Build history of the part. All positions in model axes, mm. Face numbers are marked on the shaded views. A direction names the side the tool comes from. Coordinates: 2 decimals unless noted, no trailing zeros. Loops run counter-clockwise (first coordinate to the right, second up) from the corner with the lowest first, then second, coordinate; pieces in that order, holes last. Notation, with made-up numbers: (-7, 37.25) - (10, 37.25) arc R27 ccw to (10, 56.25) - close; hole circle Ø10 at (-13.5, -31.5). An arc over 180 degrees is marked (long way). One line per item, written item: value.
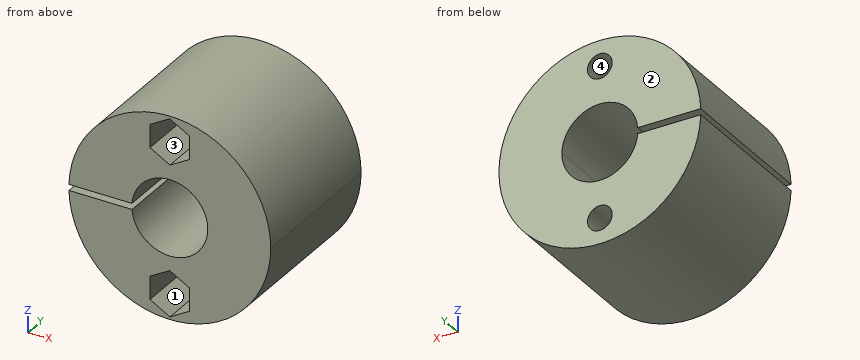
```python
from build123d import *

# Parameters (mm, degrees)
BOSS_EXTRUDE2_DEPTH = 50
CUT_EXTRUDE1_REACH  = 70.88
SKETCH3_R           = 4.1
CUT_EXTRUDE2_DEPTH  = 30


with BuildPart() as part:
    # Sketch2 → Boss-Extrude2 (new body)
    with BuildSketch(Plane(origin=(0, 0, 0), x_dir=(1, 0, 0), z_dir=(0, 1, 0))):
        with BuildLine():
            ThreePointArc((12.6, 0), (0.500394765, -12.590059773), (-12.560254774, -1))
            Line((-12.560254774, -1), (-33.485071301, -1))
            ThreePointArc((-33.485071301, -1), (0.500055713, -33.496267617), (33.5, 0))
            ThreePointArc((33.5, 0), (0.500055713, 33.496267617), (-33.485071301, 1))
            Line((-33.485071301, 1), (-12.560254774, 1))
            ThreePointArc((-12.560254774, 1), (0.500394765, 12.590059773), (12.6, 0))
        make_face()
    extrude(amount=BOSS_EXTRUDE2_DEPTH)

    # Sketch3 → Cut-Extrude1 (cut, up to next)
    with BuildSketch(Plane.XZ, mode=Mode.PRIVATE) as cut_extrude1_sk1:
        with Locations(Location((0, 25, 0), (0, 0, 270))):
            Circle(SKETCH3_R)
    cut_extrude1_tool1 = extrude(cut_extrude1_sk1.sketch, amount=-CUT_EXTRUDE1_REACH, mode=Mode.PRIVATE) & part.part
    # Sketch3 → Cut-Extrude1 (cut, up to next)
    with BuildSketch(Plane.XZ, mode=Mode.PRIVATE) as cut_extrude1_sk2:
        with Locations(Location((0, -25, 0), (0, 0, 270))):
            Circle(SKETCH3_R)
    cut_extrude1_tool2 = extrude(cut_extrude1_sk2.sketch, amount=-CUT_EXTRUDE1_REACH, mode=Mode.PRIVATE) & part.part
    add(cut_extrude1_tool1.solids().sort_by_distance((0, 0, 25))[0], mode=Mode.SUBTRACT)
    add(cut_extrude1_tool2.solids().sort_by_distance((0, 0, -25))[0], mode=Mode.SUBTRACT)

    # Sketch8 → Cut-Extrude2 (cut)
    with BuildSketch(Plane.XZ):
        Polygon((6.618426782, 21.22158407), (6.581417572, 28.842517761), (-0.03700921, 32.620933691), (-6.618426782, 28.77841593), (-6.581417572, 21.157482239), (0.03700921, 17.379066309), align=None)
        Polygon((6.618426782, -28.77841593), (6.581417572, -21.157482239), (-0.03700921, -17.379066309), (-6.618426782, -21.22158407), (-6.581417572, -28.842517761), (0.03700921, -32.620933691), align=None)
    extrude(amount=-CUT_EXTRUDE2_DEPTH, mode=Mode.SUBTRACT)


solid = part.part
```
Item 1: Cut at D-D, the plane z = 19. Write the cut outline in (x, y), then the cut area to 3 significant figures.
Check result:
outline: (-27.59, 0) - (-2.8, 0) - (-2.8, 30) - (2.81, 30) - (2.81, 0) - (27.59, 0) - (27.59, 50) - (-27.59, 50) - close
area: 2,590 mm^2
Item 2: Drop flat-ended pins along their axis: P1, Ø9.5, axis at x = 0, z = 25, coming from the -Y side; P2, Ø4, axis at y = 9, z = -4.5, coming from the +X side; P3, Ø6.5, axis at x = -19.5, y = 14, coming from the +Z side. Give the stop position or say it passes through.
Check result:
P1: stops at y = 30
P2: stops at x = 33.41
P3: stops at z = 29.29
Item 3: Tool access for the marked faces 3 and 4: list every direction of +Z, -Z, +X, -X, +Y, -Y with a clear straight run to the whole face (end or side of a thin tool).
Check result:
face 3: -Y
face 4: +Y, -Y
Item 4: Cut at B-B, the plane x = 9. Write the cut outline in (y, z).
Check result:
outline: (0, -32.27) - (50, -32.27) - (50, -8.82) - (0, -8.82) - close; (0, 8.82) - (50, 8.82) - (50, 32.27) - (0, 32.27) - close
Item 5: Pull direction X, two halves, no side cores. Call the marked faces 1 and 2: released by +X, released by -X, zero draft, split by the parting line, or undercut.
Check result:
face 1: undercut
face 2: zero draft
Item 6: Cut at C-C, the plane z = -11. Write the cut outline in (x, y), then the cut area to 3 significant figures.
Check result:
outline: (-31.64, 0) - (-6.14, 0) - (-6.14, 50) - (-31.64, 50) - close; (6.14, 0) - (31.64, 0) - (31.64, 50) - (6.14, 50) - close
area: 2,550 mm^2
Item 7: Cut at A-A, the plane y = 45. Write the cut outline in (x, z).
Check result:
outline: (-33.49, -1) arc R33.5 ccw (long way) to (-33.49, 1) - (-12.56, 1) arc R12.6 cw (long way) to (-12.56, -1) - close; hole circle Ø8.2 at (0, -25); hole circle Ø8.2 at (0, 25)
Item 8: Probe probe 1 along Z at (x, y) = (1.5, 5); probe 2 along X at (y, z) = (37.25, 25); probe 3 along X at (y, z) = (46, 21.5). List the from-to ranges inside material, lowest first. Write a range as from..to.
Check result:
probe 1: z = -33.47..-31.77, -18.26..-12.51, 12.51..18.23, 31.74..33.47
probe 2: x = -22.3..-4.1, 4.1..22.3
probe 3: x = -25.69..-2.14, 2.14..25.69
